Input: part model. Units: mm. Frame: model coordinates. Face numbers are marked on the shaded views. A direction names the side the tool comes from. Round coordinates to 2 decimals unless told otherwise and drop trailing zeros. Write each loop counter-clockwise with the first axis right and the second up, starting at its lowest first coordinate (ties: lowest second). Pieces come first, ordered by that corner, then holes. Notation, with made-up numbers: (35.5, -15) -> (57.5, -15) arc R23 cw to (57.5, 7) -> close; hole circle Ø9 at (26, -27). An arc over 180 degrees is marked (long way). Write item = value, one per line.
```python
from build123d import *

# Parameters (mm, degrees)
BOSS_EXTRUDE1_DEPTH     = 32.5
CUT_EXTRUDE1_DEPTH      = 65.662585782
CUT_EXTRUDE1_DEPTH_BACK = 65.662585782
SKETCH2_R               = 5.9
CUT_EXTRUDE2_DEPTH      = 58.282196244
CUT_EXTRUDE2_DEPTH_BACK = 58.282196244
SKETCH3_R               = 1.5
CUT_EXTRUDE3_DEPTH      = 58.282196244
CUT_EXTRUDE3_DEPTH_BACK = 58.282196244
SKETCH4_R               = 1.5
CUT_EXTRUDE4_DEPTH      = 2.5
CUT_EXTRUDE5_DEPTH      = 56.652942478
CUT_EXTRUDE5_DEPTH_BACK = 56.652942478
FILLET1_R               = 10


with BuildPart() as part:
    # Sketch1 → Boss-Extrude1 (new, symmetric)
    with BuildSketch(Plane.XY):
        with BuildLine():
            Line((-40, 0), (-40, 4))
            Line((-40, 4), (-20, 4))
            ThreePointArc((-20, 4), (-12.928932188, 6.928932188), (-10, 14))
            Line((-10, 14), (-10, 25))
            Line((-10, 25), (10, 25))
            Line((10, 25), (10, 14))
            Line((10, 14), (10, 0))
            Line((10, 0), (-40, 0))
        make_face()
    extrude(amount=BOSS_EXTRUDE1_DEPTH, both=True)

    # Sketch2 → Cut-Extrude1 (cut, two sides: drawn at the far end of the back side and taken through both)
    with BuildSketch(Plane(origin=(10, 0, 0), x_dir=(0, 0, -1), z_dir=(1, 0, 0)).offset(-CUT_EXTRUDE1_DEPTH_BACK)):
        with Locations(Location((-17.5, 15, 0), (0, 0, 350.241743405))):
            Circle(SKETCH2_R)
        with Locations(Location((17.5, 15, 0), (0, 0, 350.241743405))):
            Circle(SKETCH2_R)
    extrude(amount=CUT_EXTRUDE1_DEPTH + CUT_EXTRUDE1_DEPTH_BACK, mode=Mode.SUBTRACT)

    # Sketch3 → Cut-Extrude2 (cut, two sides: drawn at the far end of the back side and taken through both)
    with BuildSketch(Plane.XZ.offset(-CUT_EXTRUDE2_DEPTH_BACK)):
        with Locations((-35, 12)):
            Circle(SKETCH3_R)
        with Locations((-35, -12)):
            Circle(SKETCH3_R)
    extrude(amount=CUT_EXTRUDE2_DEPTH + CUT_EXTRUDE2_DEPTH_BACK, mode=Mode.SUBTRACT)

    # Sketch4 → Cut-Extrude3 (cut, two sides: drawn at the far end of the back side and taken through both)
    with BuildSketch(Plane(origin=(0, 25, 0), x_dir=(1, 0, 0), z_dir=(0, 1, 0)).offset(-CUT_EXTRUDE3_DEPTH_BACK)):
        with Locations(Location((0, 0, 0), (0, 0, 270))):
            Circle(SKETCH4_R)
    extrude(amount=CUT_EXTRUDE3_DEPTH + CUT_EXTRUDE3_DEPTH_BACK, mode=Mode.SUBTRACT)

    # Sketch5 → Cut-Extrude4 (cut)
    with BuildSketch(Plane(origin=(0, 4, 0), x_dir=(1, 0, 0), z_dir=(0, 1, 0))):
        Polygon((-32.401923789, -10.5), (-35, -9), (-37.598076211, -10.5), (-37.598076211, -13.5), (-35, -15), (-32.401923789, -13.5), align=None)
        Polygon((-32.401923789, 10.5), (-32.401923789, 13.5), (-35, 15), (-37.598076211, 13.5), (-37.598076211, 10.5), (-35, 9), align=None)
    extrude(amount=-CUT_EXTRUDE4_DEPTH, mode=Mode.SUBTRACT)

    # Sketch6 → Cut-Extrude5 (cut, two sides: drawn at the far end of the back side and taken through both)
    with BuildSketch(Plane(origin=(0, 4, 0), x_dir=(1, 0, 0), z_dir=(0, 1, 0)).offset(-CUT_EXTRUDE5_DEPTH_BACK)):
        Polygon((-20, -32.5), (-40, -24), (-40, -32.5), align=None)
        Polygon((-20, 32.5), (-40, 24), (-40, 32.5), align=None)
    extrude(amount=CUT_EXTRUDE5_DEPTH + CUT_EXTRUDE5_DEPTH_BACK, mode=Mode.SUBTRACT)

    # Fillet1
    fillet1_edges = [part.edges().sort_by_distance(p)[0] for p in [
        (-40, 2, 24),
        (-40, 2, -24),
    ]]
    fillet(fillet1_edges, radius=FILLET1_R)


solid = part.part
```
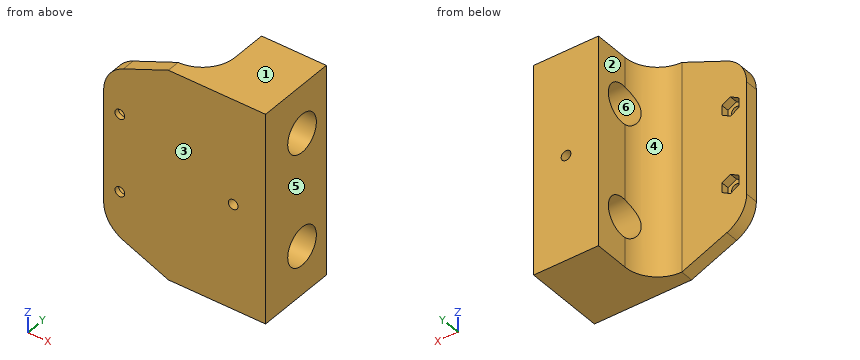
1) Cut plane A-A (z = 0). Return the cut outline in (x, y).
Solutions:
outline = (-40, 0) -> (-1.5, 0) -> (-1.5, 25) -> (-10, 25) -> (-10, 14) arc R10 cw to (-20, 4) -> (-40, 4) -> close; (1.5, 0) -> (10, 0) -> (10, 25) -> (1.5, 25) -> close
2) First-contact query: P1, Ø7, axis at y = 15, z = 17.5, coming from the +X side; P2, Ø4, axis at x = -35, z = 12, coming from the +Y side; P3, Ø10, axis at x = -29.5, z = 5, coming from the +Y side; P4, Ø12, axis at x = -23.5, z = 11.5, coming from the +Y side. Flat tips, straight axial feed; report the tip coordinate or a pass-through.
Solutions:
P1 = through
P2 = 1.5
P3 = 4
P4 = 4.32
3) Line query: L1, parallel to X at y = 0.7, z = -12; L2, parallel to Y at x = -4.5, z = -17.5; L3, parallel to Z at x = -36.5, y = 2.5. Output: solid intervals per line, ascending. Write a range as from..to.
Solutions:
L1 = -40..-36.5, -33.5..10
L2 = 0..9.1, 20.9..25
L3 = -24.98..-14.13, -9.87..9.87, 14.13..24.98
4) Cut plane D-D (y = 19). Return the cut outline in (x, z).
Solutions:
outline = (-10, -32.5) -> (10, -32.5) -> (10, -21.84) -> (-10, -21.84) -> close; (-10, -13.16) -> (10, -13.16) -> (10, 13.16) -> (-10, 13.16) -> close; (-10, 21.84) -> (10, 21.84) -> (10, 32.5) -> (-10, 32.5) -> close; hole circle Ø3 at (0, 0)
5) Cut plane B-B (y = 11.75). Return the cut outline in (x, z).
Solutions:
outline = (-10.26, -32.5) -> (10, -32.5) -> (10, -22.42) -> (-10.26, -22.42) -> close; (-10.26, -12.58) -> (10, -12.58) -> (10, 12.58) -> (-10.26, 12.58) -> close; (-10.26, 22.42) -> (10, 22.42) -> (10, 32.5) -> (-10.26, 32.5) -> close; hole circle Ø3 at (0, 0)
6) Access query for the marked faces 1 and 2. Directions: +Z, -Z, +X, -X, +Y, -Y. A direction counts if a zero-diameter tool reaches every point of the face in a straight line with its end or side. Return the directions, or none.
Solutions:
face_1 = +Z, +X, -X, +Y, -Y
face_2 = +Z, -Z, -X, +Y
7) Draft query along Y for the marked faces 3, 4, 5 and 6. Return one class per face: +Y half, -Y half, draft (parallel to the pull), parting line (faces both ways), or undercut.
Solutions:
face_3 = -Y half
face_4 = +Y half
face_5 = draft
face_6 = undercut
8) Cut plane C-C (x = 5). Return the cut outline in (y, z).
Solutions:
outline = (0, -32.5) -> (25, -32.5) -> (25, 32.5) -> (0, 32.5) -> close; hole circle Ø11.8 at (15, -17.5); hole circle Ø11.8 at (15, 17.5)
